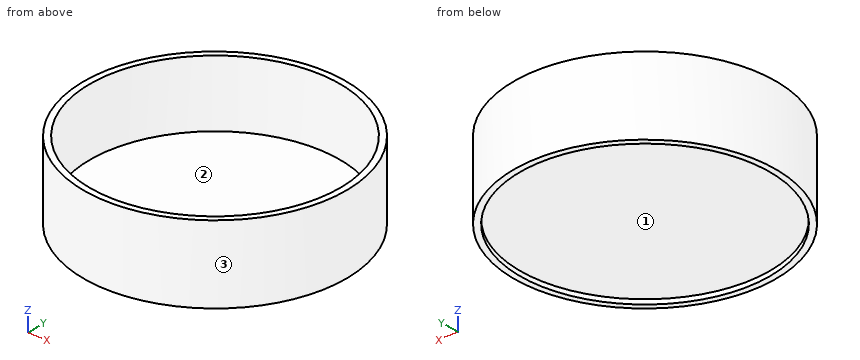
from build123d import *

# Parameters (mm, degrees)
F0_R     = 42.130231
F1_DEPTH = 2
F3_R     = 42.5
F3_R_2   = 40.5
F4_DEPTH = 25


with BuildPart() as f1:
    # F0 (on Top) → F1 (new body)
    with BuildSketch(Plane.XY):
        Circle(F0_R)
    extrude(amount=F1_DEPTH)


with BuildPart() as f1_1:
    # F2: moved
    add(f1.part.moved(Location((0, 0, 1.5))))

    # F3 (on Top) → F4 (join)
    with BuildSketch(Plane.XY):
        Circle(F3_R)
        Circle(F3_R_2, mode=Mode.SUBTRACT)
    extrude(amount=F4_DEPTH)


solid = f1_1.part
The model under review builds one solid part; all positions refer to its coordinate system, in mm. Face numbers are marked on the shaded views. Round coordinates to 2 decimals unless told otherwise and drop trailing zeros. Order: outer loops, then holes, each group sorted by start corner. A loop starts at its lowest first (then second) coordinate and runs counter-clockwise, first axis right, second up. Notation, with made-up numbers: (-33.5, -2.75) -> (-1.5, -2.75) arc R30 cw to (-1.5, 31.25) -> close; hole circle Ø8 at (5.25, 33.25). An arc over 180 degrees is marked (long way). Write item = value, one per line. Start each with the question number.
Item 1: Consider section A-A on x = 0. Write out the cut boundary in (y, z), plus the area to 3 significant figures.
Item 2: Consider section B-B on z = 16.5. Write out the cut boundary in (x, y), plus the area to 3 significant figures.
Item 3: For line 1 along Y through (x, z) = (0, 9); line 2 along Z through (x, y) = (-10, -6.5); line 3 along X through (y, z) = (-22.5, 18.75), list the stretches that pass through material, from the lowest coordinate up.
Item 4: Mouldability with a two-part tool opening along Y and no side actions: class the marked faces 1, 2 and 3 as released by +Y, released by -Y, zero draft, split by the parting line, or undercut.
Item 5: Clearance check with flat-ended pins moving along their axes: pin 1 Ø4 at (x, y) = (3.5, -7) entering from -Z; pin 2 Ø10 at (x, z) = (20.5, 17.5) entering from +Y; pin 3 Ø8 at (x, y) = (-27.5, -23) entering from +Z. State where each tip first meets the part, or that it passes through.
Conclusion:
q1.outline = (-42.5, 0) -> (-40.5, 0) -> (-40.5, 1.5) -> (40.5, 1.5) -> (40.5, 0) -> (42.5, 0) -> (42.5, 25) -> (40.5, 25) -> (40.5, 3.5) -> (-40.5, 3.5) -> (-40.5, 25) -> (-42.5, 25) -> close
q1.area = 262 mm2
q2.outline = circle Ø85 at (0, 0); hole circle Ø81 at (0, 0)
q2.area = 522 mm2
q3.line_1 = -42.5 to -40.5, 40.5 to 42.5
q3.line_2 = 1.5 to 3.5
q3.line_3 = -36.06 to -33.67, 33.67 to 36.06
q4.face_1 = undercut
q4.face_2 = undercut
q4.face_3 = split by the parting line
q5.pin_1 = 1.5
q5.pin_2 = 39.57
q5.pin_3 = 3.5
